```python
from build123d import *

# Parameters (mm, degrees)
BOSS_EXTRUDE1_DEPTH = 18
SKETCH2_R           = 1.75
CUT_EXTRUDE1_DEPTH  = 32.5
CUT_EXTRUDE2_DEPTH  = 1
CUT_EXTRUDE3_DEPTH  = 5


with BuildPart() as part:
    # Sketch1 → Boss-Extrude1 (new body)
    with BuildSketch(Plane(origin=(0, 0, 0), x_dir=(1, 0, 0), z_dir=(0, 1, 0))):
        with BuildLine():
            Line((-12.998275301, 32.528571429), (-29.998275301, 32.528571429))
            Line((-29.998275301, 32.528571429), (-29.998275301, 19.047432641))
            ThreePointArc((-29.998275301, 19.047432641), (-21.855641496, 22.757647896), (-12.998275301, 24.028571429))
            Line((-12.998275301, 24.028571429), (-12.998275301, 32.528571429))
        make_face()
        with BuildLine():
            ThreePointArc((-12.998275301, 24.028571429), (-21.855641496, 22.757647896), (-29.998275301, 19.047432641))
            ThreePointArc((-29.998275301, 19.047432641), (-44.498275301, -7.471428571), (-29.998275301, -33.990289784))
            ThreePointArc((-29.998275301, -33.990289784), (-21.855641496, -37.700505039), (-12.998275301, -38.971428571))
            Line((-12.998275301, -38.971428571), (-12.998275301, -31.971428571))
            ThreePointArc((-12.998275301, -31.971428571), (-37.498275301, -7.471428571), (-12.998275301, 17.028571429))
            Line((-12.998275301, 17.028571429), (-12.998275301, 24.028571429))
        make_face()
        with BuildLine():
            Line((-29.998275301, -33.990289784), (-29.998275301, -47.471428571))
            Line((-29.998275301, -47.471428571), (-12.998275301, -47.471428571))
            Line((-12.998275301, -47.471428571), (-12.998275301, -38.971428571))
            ThreePointArc((-12.998275301, -38.971428571), (-21.855641496, -37.700505039), (-29.998275301, -33.990289784))
        make_face()
    extrude(amount=BOSS_EXTRUDE1_DEPTH)

    # Sketch2 → Cut-Extrude1 (cut, through all)
    with BuildSketch(Plane(origin=(-12.998275301, 0, 0), x_dir=(0, 0, -1), z_dir=(1, 0, 0))):
        with Locations((-42.471428571, 5.25)):
            Circle(SKETCH2_R)
        with Locations((27.528571429, 5.25)):
            Circle(SKETCH2_R)
    extrude(amount=-CUT_EXTRUDE1_DEPTH, mode=Mode.SUBTRACT)

    # Sketch3 → Cut-Extrude2 (cut)
    with BuildSketch(Plane(origin=(-12.998275301, 0, 0), x_dir=(0, 0, -1), z_dir=(1, 0, 0))):
        Polygon((-41.872123333, 15.051635835), (-39.29413188, 15.051635835), (-39.29413188, 14.10184951), (-40.922337009, 14.10184951), (-40.922337009, 13.084221305), (-39.29413188, 13.084221305), (-39.29413188, 12.13443498), (-40.922337009, 12.13443498), (-40.922337009, 9.759969168), (-41.872123333, 9.759969168), align=None)
        with BuildLine():
            Line((-37.768749602, 15.051635835), (-35.359302821, 15.051635835))
            Line((-35.359302821, 15.051635835), (-35.359302821, 14.16969139))
            Line((-35.359302821, 14.16969139), (-37.016128742, 14.16969139))
            Line((-37.016128742, 14.16969139), (-37.222834471, 13.169023655))
            add(Edge.make_bspline(
                [(-37.222834471, 13.169023655), (-37.194667857, 13.176868413), (-37.139117506, 13.192339887), (-37.055430833, 13.207855818), (-36.974326785, 13.217912751), (-36.921106803, 13.219254212), (-36.895285393, 13.219905065)],
                knots=[0, 0, 0, 0, 8.7675e-05, 0.000172914, 0.000255092, 0.000332539, 0.000332539, 0.000332539, 0.000332539], degree=3))
            add(Edge.make_bspline(
                [(-36.895285393, 13.219905065), (-36.839017834, 13.218615727), (-36.728102081, 13.216074157), (-36.56584641, 13.191946365), (-36.410477019, 13.153945825), (-36.262469357, 13.099749215), (-36.121968006, 13.029210927), (-35.988802653, 12.943879371), (-35.862809858, 12.843604675), (-35.746227784, 12.728324059), (-35.639107304, 12.601743331), (-35.545972157, 12.464832881), (-35.466428929, 12.319544917), (-35.403162996, 12.164976334), (-35.353228128, 12.002097925), (-35.317144077, 11.830805314), (-35.295805775, 11.650895492), (-35.292928436, 11.528155884), (-35.29146094, 11.465556441)],
                knots=[0, 0, 0, 0, 0.000168708, 0.00033256, 0.000490931, 0.00064788, 0.00080432, 0.000961637, 0.001121557, 0.001286466, 0.001452728, 0.001618259, 0.001782383, 0.001948726, 0.00211839, 0.002292819, 0.002473214, 0.002660986, 0.002660986, 0.002660986, 0.002660986], degree=3))
            add(Edge.make_bspline(
                [(-35.29146094, 11.465556441), (-35.293254243, 11.402246349), (-35.296792955, 11.277317032), (-35.319879804, 11.093626745), (-35.360628507, 10.917692919), (-35.416600928, 10.749044582), (-35.490341009, 10.588921261), (-35.579023549, 10.435664197), (-35.684147931, 10.290410967), (-35.804682523, 10.154650595), (-35.935719436, 10.030563008), (-36.075242816, 9.921402921), (-36.22227247, 9.829545591), (-36.376811944, 9.75530934), (-36.537974597, 9.696574939), (-36.705809344, 9.653819098), (-36.881131839, 9.629301), (-37.000153034, 9.625975643), (-37.060649976, 9.624285407)],
                knots=[0, 0, 0, 0, 0.000189935, 0.000374797, 0.00055428, 0.000730936, 0.00090692, 0.001082188, 0.001261361, 0.001443849, 0.001626066, 0.00180206, 0.001974425, 0.002145103, 0.002315455, 0.002488223, 0.002663769, 0.002845232, 0.002845232, 0.002845232, 0.002845232], degree=3))
            add(Edge.make_bspline(
                [(-37.060649976, 9.624285407), (-37.11475059, 9.625668125), (-37.221448324, 9.628395135), (-37.378609401, 9.645156773), (-37.530130131, 9.674791505), (-37.675206106, 9.717680636), (-37.815363767, 9.770467365), (-37.94898285, 9.836487145), (-38.076797617, 9.914482872), (-38.198445122, 10.00303112), (-38.311948765, 10.102777287), (-38.415542863, 10.211966653), (-38.509854588, 10.329222939), (-38.592865818, 10.455992731), (-38.664316336, 10.592088734), (-38.727680113, 10.735907025), (-38.779543999, 10.888949526), (-38.805863427, 10.99504709), (-38.819238718, 11.048964895)],
                knots=[0, 0, 0, 0, 0.000162309, 0.000320108, 0.00047353, 0.000624818, 0.000773452, 0.00092231, 0.001071202, 0.001222162, 0.001373137, 0.001523844, 0.001673169, 0.001823995, 0.001977637, 0.002133811, 0.002295051, 0.002461661, 0.002461661, 0.002461661, 0.002461661], degree=3))
            Line((-38.819238718, 11.048964895), (-37.733768633, 11.048964895))
            add(Edge.make_bspline(
                [(-37.733768633, 11.048964895), (-37.713926213, 11.011602052), (-37.675364736, 10.938991631), (-37.60201228, 10.842590387), (-37.519898863, 10.760383548), (-37.429765192, 10.691567935), (-37.331027257, 10.640012448), (-37.227708443, 10.600915152), (-37.118510798, 10.578322273), (-37.044142381, 10.575497939), (-37.006588478, 10.574071732)],
                knots=[0, 0, 0, 0, 0.000126748, 0.00024632, 0.000361751, 0.000474538, 0.000585031, 0.000694707, 0.000805098, 0.000917705, 0.000917705, 0.000917705, 0.000917705], degree=3))
            add(Edge.make_bspline(
                [(-37.006588478, 10.574071732), (-36.980413911, 10.575056541), (-36.92891501, 10.576994168), (-36.853039524, 10.587244701), (-36.780613038, 10.60665898), (-36.71109708, 10.633543242), (-36.644304912, 10.667070955), (-36.581194023, 10.709397506), (-36.520666397, 10.758116937), (-36.46364351, 10.814022648), (-36.411997211, 10.876344513), (-36.366709056, 10.943313604), (-36.3262152, 11.013441856), (-36.296220781, 11.089507223), (-36.271657889, 11.169238367), (-36.253568781, 11.253236725), (-36.2427585, 11.341600399), (-36.241757757, 11.401923802), (-36.241247265, 11.43269553)],
                knots=[0, 0, 0, 0, 7.8557e-05, 0.000154562, 0.000229126, 0.000302949, 0.000377852, 0.000452822, 0.000530465, 0.000610671, 0.000691969, 0.000772824, 0.000853029, 0.000934327, 0.001017484, 0.001103143, 0.001191762, 0.001284039, 0.001284039, 0.001284039, 0.001284039], degree=3))
            add(Edge.make_bspline(
                [(-36.241247265, 11.43269553), (-36.24183975, 11.462752977), (-36.242993035, 11.521260526), (-36.252533243, 11.607170565), (-36.269600491, 11.688683645), (-36.292854763, 11.766424094), (-36.322623008, 11.839919836), (-36.359001793, 11.909608351), (-36.402146532, 11.975137391), (-36.452288859, 12.035172848), (-36.505760122, 12.090239076), (-36.56320544, 12.138399561), (-36.624107261, 12.178369419), (-36.686573137, 12.213264269), (-36.753096479, 12.238659979), (-36.822181447, 12.256149068), (-36.893755387, 12.268981858), (-36.942574418, 12.269735832), (-36.967367391, 12.270118741)],
                knots=[0, 0, 0, 0, 9.0159e-05, 0.000175496, 0.000258862, 0.000339682, 0.000418616, 0.000496375, 0.000575167, 0.000653481, 0.000730688, 0.0008052, 0.000877818, 0.000948966, 0.00101944, 0.00109066, 0.001162633, 0.001236903, 0.001236903, 0.001236903, 0.001236903], degree=3))
            add(Edge.make_bspline(
                [(-36.967367391, 12.270118741), (-36.994298321, 12.269096861), (-37.048273682, 12.267048796), (-37.12846756, 12.250384238), (-37.207694523, 12.22341473), (-37.286395154, 12.186206021), (-37.363788212, 12.13751156), (-37.44191614, 12.080398541), (-37.518163827, 12.010717161), (-37.566644228, 11.95881831), (-37.591724696, 11.931969368)],
                knots=[0, 0, 0, 0, 8.0736e-05, 0.000161813, 0.000244611, 0.000331384, 0.000422288, 0.00051854, 0.000621363, 0.000731571, 0.000731571, 0.000731571, 0.000731571], degree=3))
            Line((-37.591724696, 11.931969368), (-38.390986848, 12.115354451))
            Line((-38.390986848, 12.115354451), (-37.768749602, 15.051635835))
        make_face()
    extrude(amount=-CUT_EXTRUDE2_DEPTH, mode=Mode.SUBTRACT)

    # Sketch4 → Cut-Extrude3 (cut)
    with BuildSketch(Plane.ZY.offset(29.998275301)):
        Polygon((-25.65109293, 2.689061145), (-24.371994073, 5.595474648), (-26.249472572, 8.156413503), (-29.406049928, 7.810938855), (-30.685148784, 4.904525352), (-28.807670285, 2.343586497), align=None)
        Polygon((44.048403814, 2.493828304), (45.646830899, 5.237614774), (44.069855656, 7.993786469), (40.894453329, 8.006171696), (39.296026244, 5.262385226), (40.873001487, 2.506213531), align=None)
    extrude(amount=-CUT_EXTRUDE3_DEPTH, mode=Mode.SUBTRACT)


solid = part.part
```
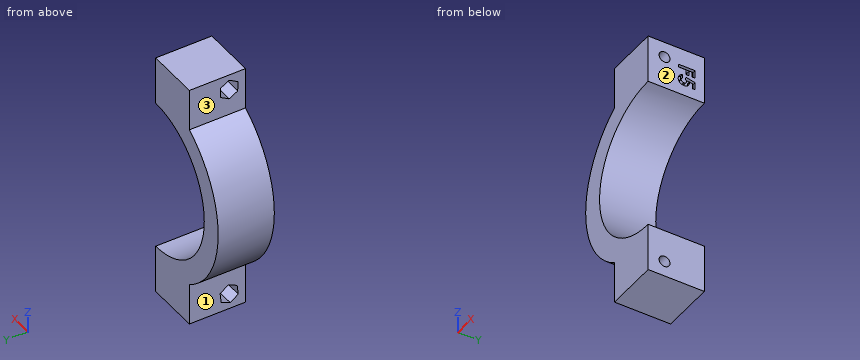
Geometry check sheet. Reference: the model listing, model coordinates, mm. Face numbers are marked on the shaded views. A direction names the side the tool comes from. Round coordinates to 2 decimals unless told otherwise and drop trailing zeros. Order: outer loops, then holes, each group sorted by start corner. A loop starts at its lowest first (then second) coordinate and runs counter-clockwise, first axis right, second up. Notation, with made-up numbers: (31.5, -7) - (50.5, -7) arc R32 ccw to (50.5, 22) - close; hole circle Ø11 at (43.25, 46.25). An arc over 180 degrees is marked (long way). Use a Markdown table: item, result. Add a question column.
(1) Depth check by flat-ended pin: pin 1 (6 mm diameter, centred on y = 6.5, z = 43.5, fed in from -X). Enter the tip coordinate at first touch or a pass-through.
(2) Material ranges on line 1 along Z through (x, y) = (-13.5, 16.25); line 2 along Z through (x, y) = (-24, 3.25); line 3 along X through (y, z) = (17.25, 37.5), recorded low to high. Write a range as [from, to].
(3) Tool access check on the marked faces 1, 2 and 3. Record the directions out of +Z, -Z, +X, -X, +Y, -Y that give a thin tool (end or side, any length) a straight path to the whole face; none if there is none.
(4) Sectioned sample at C-C, the plane z = 25.5. Enter the section's corners in (x, y).
(5) Sectioned sample at B-B, the plane z = -3.5. Enter the section's corners in (x, y).
(6) Sectioned sample at A-A, the plane x = -32. Enter the section's corners in (y, z).
Answers below:
| question | item | result |
|---|---|---|
| 1 | pin 1 | x = -30 |
| 2 | line 1 | [-32.53, -17.02], [31.97, 47.47] |
| 2 | line 2 | [-32.53, -14.42], [29.36, 47.47] |
| 2 | line 3 | [-30, -13] |
| 3 | face 1 | -Z, -X, +Y, -Y |
| 3 | face 2 | +Z, -Z, +X, +Y, -Y |
| 3 | face 3 | +Z, -X, +Y, -Y |
| 4 | outline | (-38.83, 0) - (-29.59, 0) - (-29.59, 18) - (-38.83, 18) - close |
| 5 | outline | (-42.53, 0) - (-34.9, 0) - (-34.9, 18) - (-42.53, 18) - close |
| 6 | outline | (0, -17.65) - (18, -17.65) - (18, -7.99) - (0, -7.99) - close; (0, 22.94) - (18, 22.94) - (18, 32.59) - (0, 32.59) - close |
